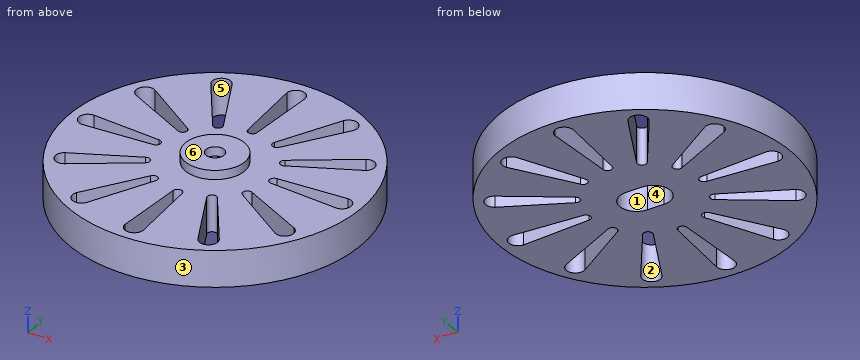
```python
from build123d import *

# Parameters (mm, degrees)
ESQUISSE1_R                  = 16
BOSS_EXTRU_1_DEPTH           = 4
ESQUISSE2_R                  = 3.25
BOSS_EXTRU_2_DEPTH           = 1
ENL_V_MAT_EXTRU_1_REACH      = 25.173
ESQUISSE3_R                  = 1
ENL_V_MAT_EXTRU_2_DEPTH      = 4
ENL_V_MAT_EXTRU_4_REACH      = 25.173
R_P_TITION_CIRCULAIRE1_COUNT = 12


with BuildPart() as part:
    # Esquisse1 → Boss.-Extru.1 (new body)
    with BuildSketch(Plane.XY):
        Circle(ESQUISSE1_R)
    extrude(amount=BOSS_EXTRU_1_DEPTH)

    # Esquisse2 → Boss.-Extru.2 (add)
    with BuildSketch(Plane.XY.offset(4)):
        Circle(ESQUISSE2_R)
    extrude(amount=BOSS_EXTRU_2_DEPTH)

    # Esquisse3 → Enlèv. mat.-Extru.1 (cut, up to next)
    with BuildSketch(Plane.XY.offset(5), mode=Mode.PRIVATE) as enl_v_mat_extru_1_sk1:
        Circle(ESQUISSE3_R)
    enl_v_mat_extru_1_tool1 = extrude(enl_v_mat_extru_1_sk1.sketch, amount=-ENL_V_MAT_EXTRU_1_REACH, mode=Mode.PRIVATE) & part.part
    add(enl_v_mat_extru_1_tool1.solids().sort_by_distance((0, 0, 5))[0], mode=Mode.SUBTRACT)

    # Esquisse4 → Enlèv. mat.-Extru.2 (cut)
    with BuildSketch(Plane(origin=(0, 0, 0), x_dir=(-1, 0, 0), z_dir=(0, 0, -1))):
        with BuildLine():
            Line((-0.925, 1.85), (0.925, 1.85))
            ThreePointArc((0.925, 1.85), (2.775, 0), (0.925, -1.85))
            Line((0.925, -1.85), (-0.925, -1.85))
            ThreePointArc((-0.925, -1.85), (-2.775, 0), (-0.925, 1.85))
        make_face()
    extrude(amount=-ENL_V_MAT_EXTRU_2_DEPTH, mode=Mode.SUBTRACT)

    # Esquisse5 → Enlèv. mat.-Extru.4 (cut, up to next)
    with BuildSketch(Plane(origin=(0, 0, 0), x_dir=(-1, 0, 0), z_dir=(0, 0, -1)), mode=Mode.PRIVATE) as enl_v_mat_extru_4_sk1:
        with BuildLine():
            Line((6.5, 0.5), (14, 1))
            ThreePointArc((14, 1), (15, 0), (14, -1))
            Line((14, -1), (6.5, -0.5))
            ThreePointArc((6.5, -0.5), (6, 0), (6.5, 0.5))
        make_face()
    enl_v_mat_extru_4_tool1 = extrude(enl_v_mat_extru_4_sk1.sketch, amount=-ENL_V_MAT_EXTRU_4_REACH, mode=Mode.PRIVATE) & part.part
    enl_v_mat_extru_4 = enl_v_mat_extru_4_tool1.solids().sort_by_distance((-10.983243, 0, 0))[0]
    add(enl_v_mat_extru_4, mode=Mode.SUBTRACT)

    # Répétition circulaire1: Enlèv. mat.-Extru.4 ×12 about axis
    r_p_tition_circulaire1_axis = Axis((0, 0, 0), (0, 0, 1))
    for i in range(1, R_P_TITION_CIRCULAIRE1_COUNT):
        add(enl_v_mat_extru_4.rotate(r_p_tition_circulaire1_axis, i * 360 / R_P_TITION_CIRCULAIRE1_COUNT), mode=Mode.SUBTRACT)


solid = part.part
```
The listing builds one solid part. Answer for the finished solid, in the listing's coordinates (mm). Face numbers are marked on the shaded views. A direction names the side the tool comes from. Give positions to 0.01 mm unless a question says otherwise; leave off trailing zeros. Order: outer loops, then holes, each group sorted by start corner. A loop starts at its lowest first (then second) coordinate and runs counter-clockwise, first axis right, second up. Notation, with made-up numbers: (75, 85.5) - (80, 85.5) arc R29 ccw to (80, 107.5) - close; hole circle Ø11 at (35.5, 53.25). An arc over 180 degrees is marked (long way). Answer in a Markdown table with one row per item. Add a question column.
Q1. Which of the six approach directions +Z, -Z, +X, -X, +Y, -Y give full straight-line access (tool end or side, diameter ignored) to the marked faces 1 and 2?
Q2. The part is cut by section A-A (x = 0). Determine the outline of the cut face in (y, z), then the cut area to 3 significant figures.
Q3. Find the intervals of material crossed by line 1 along Y through (x, z) = (0, 4.5); line 2 along X through (y, z) = (-6.5, 2.7); line 3 along X through (y, z) = (-11.5, 3.35), in increasing order. Write a range as [from, to].
Q4. The part is cut by section C-C (x = 7). Determine the outline of the cut face in (y, z), then the cut area to 3 significant figures.
Q5. For a pull along Y with two mould halves and no side action, classify the marked faces 3, 4, 5 and 6 as released by +Y, released by -Y, zero draft, split by the parting line, or undercut.
Q6. Given P1, Ø1.5, axis at y = 4.5, z = 2, coming from the -X side, flat-ended and moving along its own axis, determine where the tip first touches the part or whether it passes through.
Q7. The part is cut by section B-B (y = -4.5). Determine the outline of the cut face in (x, z), then the cut area to 3 significant figures.
Q8. The part is cut by section D-D (z = 2.1). Give the number of separate pieces and of enclosed holes in the cut face, then the cut area to 3 significant figures.
Determined:
| question | item | result |
|---|---|---|
| 1 | face 1 | -Z |
| 1 | face 2 | +Z, -Z |
| 2 | outline | (-16, 0) - (-15, 0) - (-15, 4) - (-16, 4) - close; (-6, 0) - (-1.85, 0) - (-1.85, 4) - (-1, 4) - (-1, 5) - (-3.25, 5) - (-3.25, 4) - (-6, 4) - close; (1, 4) - (1.85, 4) - (1.85, 0) - (6, 0) - (6, 4) - (3.25, 4) - (3.25, 5) - (1, 5) - close; (15, 0) - (16, 0) - (16, 4) - (15, 4) - close |
| 2 | area | 45.7 mm² |
| 3 | line 1 | y = [-3.25, -1], [1, 3.25] |
| 3 | line 2 | x = [-14.62, -12.99], [-9.58, -4.43], [-3.12, -0.5], [0.5, 3.12], [4.43, 9.58], [12.99, 14.62] |
| 3 | line 3 | x = [-11.12, -7.78], [-5.58, -0.83], [0.83, 5.58], [7.78, 11.12] |
| 4 | outline | (-14.39, 0) - (-13.12, 0) - (-13.12, 4) - (-14.39, 4) - close; (-10.33, 0) - (-4.77, 0) - (-4.77, 4) - (-10.33, 4) - close; (-3.37, 0) - (-0.53, 0) - (-0.53, 4) - (-3.37, 4) - close; (0.53, 0) - (3.37, 0) - (3.37, 4) - (0.53, 4) - close; (4.77, 0) - (10.33, 0) - (10.33, 4) - (4.77, 4) - close; (13.12, 0) - (14.39, 0) - (14.39, 4) - (13.12, 4) - close |
| 4 | area | 77.3 mm² |
| 5 | face 3 | split by the parting line |
| 5 | face 4 | undercut |
| 5 | face 5 | undercut |
| 5 | face 6 | zero draft |
| 6 | P1 | stops at x = -15.55 |
| 7 | outline | (-15.35, 0) - (-9.3, 0) - (-9.3, 4) - (-15.35, 4) - close; (-6.6, 0) - (6.6, 0) - (6.6, 4) - (-6.6, 4) - close; (9.3, 0) - (15.35, 0) - (15.35, 4) - (9.3, 4) - close |
| 7 | area | 101 mm² |
| 8 | separate pieces | 1 |
| 8 | enclosed holes | 13 |
| 8 | area | 628 mm² |
